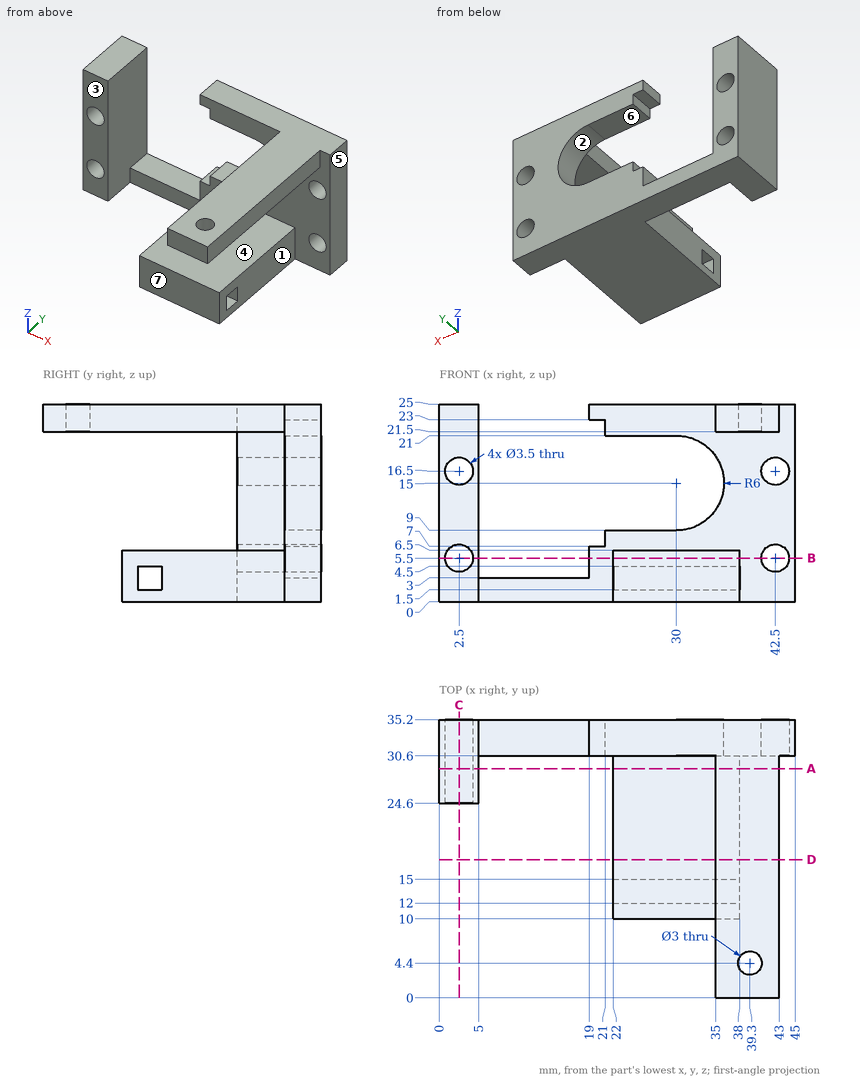
For this review, use the dimensioned drawing (mm, ordinates from the lowest corner) and the shaded views. A direction names the side the tool comes from. Coordinates: 2 decimals unless noted, no trailing zeros. Write each loop counter-clockwise with the first axis right and the second up, starting at its lowest first coordinate (ties: lowest second). Pieces come first, ordered by that corner, then holes. Notation, with made-up numbers: (-36, -37.75) - (8, -37.75) arc R29 ccw to (8, 0.25) - close; hole circle Ø7 at (30, 41.25). An arc over 180 degrees is marked (long way). Answer as a JSON object with one key per item and string values. Group by question number.
1. To check wall thickness, follow probe 1 along Z at (x, y) = (42.5, 33.9); probe 2 along X at (y, z) = (27.5, 16.5); probe 3 along Z at (x, y) = (20, 31.5). State the ranges of each line that lie inside material, in increasing order.
2. Add section D-D (y = 17.5). Give the boundary of the cut face in (x, z), plus the area to 3 significant figures.
3. Machinability: for the marked faces 1, 2, 3 and 4, which of the approach directions +Z, -Z, +X, -X, +Y, -Y give a long, thin tool a straight path to every point of the face, cutting with its end or side? Answer none if there is none.
4. Add section C-C (x = 2.5). Give the boundary of the cut face in (y, z), plus the area to 3 significant figures.
5. Clearance check with flat-ended pins moving along their axes: pin 1 Ø7 at (y, z) = (21.5, 3.5) entering from +X; pin 2 Ø2 at (y, z) = (33.5, 22.5) entering from -X; pin 3 Ø3 at (y, z) = (13.5, 22.5) entering from +X; pin 4 Ø0.9 at (x, y) = (29, 13.5) entering from +Z. State where each tip first meets the part, or that it passes through.
6. Add section B-B (z = 5.5). Give the boundary of the cut face in (x, y).
7. Add section A-A (y = 29). Give the boundary of the cut face in (x, z).
8. Mouldability with a two-part tool opening along X and no side actions: class the marked faces 5, 6 and 7 as pulls with the +X half, pulls with the -X half, needs draft (parallel to the pull), parting line crosses it, or undercut.
Findings:
{
 "1": {"probe 1": "0 to 3.75, 7.25 to 14.75, 18.25 to 25", "probe 2": "0 to 0.75, 4.25 to 5", "probe 3": "0 to 7, 23 to 25"},
 "2": {"outline": "(22, 0) - (38, 0) - (38, 6.5) - (22, 6.5) - close; (35, 21.5) - (43, 21.5) - (43, 25) - (35, 25) - close", "area": "132 mm²"},
 "3": {"face 1": "-Z, +X, -Y", "face 2": "+Y, -Y", "face 3": "+Z, -Z, -X, -Y", "face 4": "+X, -Y"},
 "4": {"outline": "(24.6, 0) - (35.2, 0) - (35.2, 3.75) - (24.6, 3.75) - close; (24.6, 7.25) - (35.2, 7.25) - (35.2, 14.75) - (24.6, 14.75) - close; (24.6, 18.25) - (35.2, 18.25) - (35.2, 25) - (24.6, 25) - close", "area": "191 mm²"},
 "5": {"pin 1": "x = 38", "pin 2": "x = 0", "pin 3": "x = 43", "pin 4": "z = 6.5"},
 "6": {"outline": "(0, 24.6) - (0.75, 24.6) - (0.75, 35.2) - (0, 35.2) - close; (4.25, 24.6) - (5, 24.6) - (5, 35.2) - (4.25, 35.2) - close; (19, 30.6) - (22, 30.6) - (22, 10) - (38, 10) - (38, 30.6) - (40.75, 30.6) - (40.75, 35.2) - (19, 35.2) - close; (44.25, 30.6) - (45, 30.6) - (45, 35.2) - (44.25, 35.2) - close"},
 "7": {"outline": "(0, 0) - (5, 0) - (5, 25) - (0, 25) - close; (22, 0) - (38, 0) - (38, 6.5) - (22, 6.5) - close; (35, 21.5) - (43, 21.5) - (43, 25) - (35, 25) - close; hole circle Ø3.5 at (2.5, 5.5); hole circle Ø3.5 at (2.5, 16.5)"},
 "8": {"face 5": "pulls with the +X half", "face 6": "undercut", "face 7": "needs draft"}
}
